from build123d import *

# Parameters (mm, degrees)
SKETCH1_R           = 12.8
BOSS_EXTRUDE2_DEPTH = 10
FILLET1_R           = 5


with BuildPart() as part:
    # Sketch1 → Boss-Extrude2 (new body)
    with BuildSketch(Plane(origin=(0, 0, 0), x_dir=(1, 0, 0), z_dir=(0, 1, 0))):
        with BuildLine():
            Line((15.087461292, -16.184019493), (15.087461292, 1.615980507))
            ThreePointArc((15.087461292, 1.615980507), (-6.93154333, 18.908753564), (-18.512538708, -6.581580106))
            Line((-18.512538708, -6.581580106), (-18.512538708, -16.184019493))
            Line((-18.512538708, -16.184019493), (15.087461292, -16.184019493))
        make_face()
        with Locations(Location((-2.712538708, 1.615980507, 0), (0, 0, 270))):
            Circle(SKETCH1_R, mode=Mode.SUBTRACT)
    extrude(amount=BOSS_EXTRUDE2_DEPTH)

    # Fillet1
    fillet1_edges = [part.edges().sort_by_distance(p)[0] for p in [
        (15.087461292, 5, 16.184019493),
        (-18.512538708, 5, 16.184019493),
    ]]
    fillet(fillet1_edges, radius=FILLET1_R)


solid = part.part
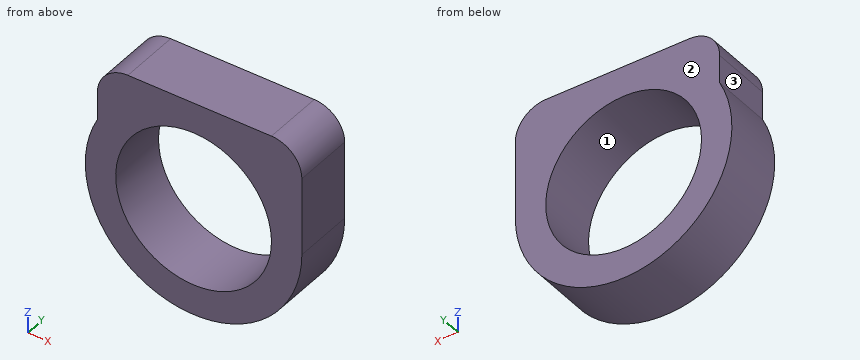
Build history of the part. All positions in model axes, mm. Face numbers are marked on the shaded views. Round coordinates to 2 decimals unless told otherwise and drop trailing zeros. Loops run counter-clockwise (first coordinate to the right, second up) from the corner with the lowest first, then second, coordinate; pieces in that order, holes last. Notation, with made-up numbers: (14.5, 48.25) -> (18.5, 48.25) arc R21 cw to (18.5, 83.25) -> close; hole circle Ø2 at (60, 34). An arc over 180 degrees is marked (long way). One line per item, written item: value. Start each with the question number.
Q1. Probe line 1 along X through (y, z) = (1, -1.5); line 2 along X through (y, z) = (9.25, 4.5); line 3 along Z through (x, y) = (6, 4.5). List the from-to ranges inside material, lowest first.
Q2. Cut at B-B on x = -12. List the corners of the cut face in (y, z), plus the area to 3 significant figures.
Q3. Two-plate mould, pull along X, no slides. Class the marked faces 1, 2 and 3: released by +X, released by -X, zero draft, split by the parting line, or undercut.
Q4. Cut at A-A on z = 7. List the corners of the cut face in (x, y).
Q5. Cut at D-D on z = 12. List the corners of the cut face in (x, y).
Q6. Drop flat-ended pins along their axis: pin 1 Ø6 at (y, z) = (7.5, -9.5) entering from +X; pin 2 Ø3.5 at (y, z) = (4, 9) entering from -X; pin 3 Ø2 at (y, z) = (6, -8) entering from -X. Give the stop position or say it passes through.
Q7. Cut at C-C on y = 7. List the corners of the cut face in (x, z).
Computed:
1. line 1: -20.51 to -15.51, 10.09 to 15.09
1. line 2: -19.43 to -13.96, 8.53 to 15.09
1. line 3: -17.14 to -10.99, 7.76 to 16.18
2. outline: (0, -16.8) -> (10, -16.8) -> (10, -10.42) -> (0, -10.42) -> close; (0, 7.19) -> (10, 7.19) -> (10, 16.18) -> (0, 16.18) -> close
2. area: 154 mm²
3. face 1: undercut
3. face 2: zero draft
3. face 3: released by -X
4. outline: (-18.51, 0) -> (-12.18, 0) -> (-12.18, 10) -> (-18.51, 10) -> close; (6.75, 0) -> (15.09, 0) -> (15.09, 10) -> (6.75, 10) -> close
5. outline: (-18.45, 0) -> (15.02, 0) -> (15.02, 10) -> (-18.45, 10) -> close
6. pin 1: x = 14.4
6. pin 2: x = -18.51
6. pin 3: x = -19.68
7. outline: (-18.51, 6.58) arc R17.8 ccw (long way) to (15.09, -1.62) -> (15.09, 11.18) arc R5 ccw to (10.09, 16.18) -> (-13.51, 16.18) arc R5 ccw to (-18.51, 11.18) -> close; hole circle Ø25.6 at (-2.71, -1.62)
